Source: three-view drawing plus pictorial views. Frame: mm from the lowest corner of the part. Coordinates: 2 decimals unless noted, no trailing zeros. Loops run counter-clockwise (first coordinate to the right, second up) from the corner with the lowest first, then second, coordinate; pieces in that order, holes last.
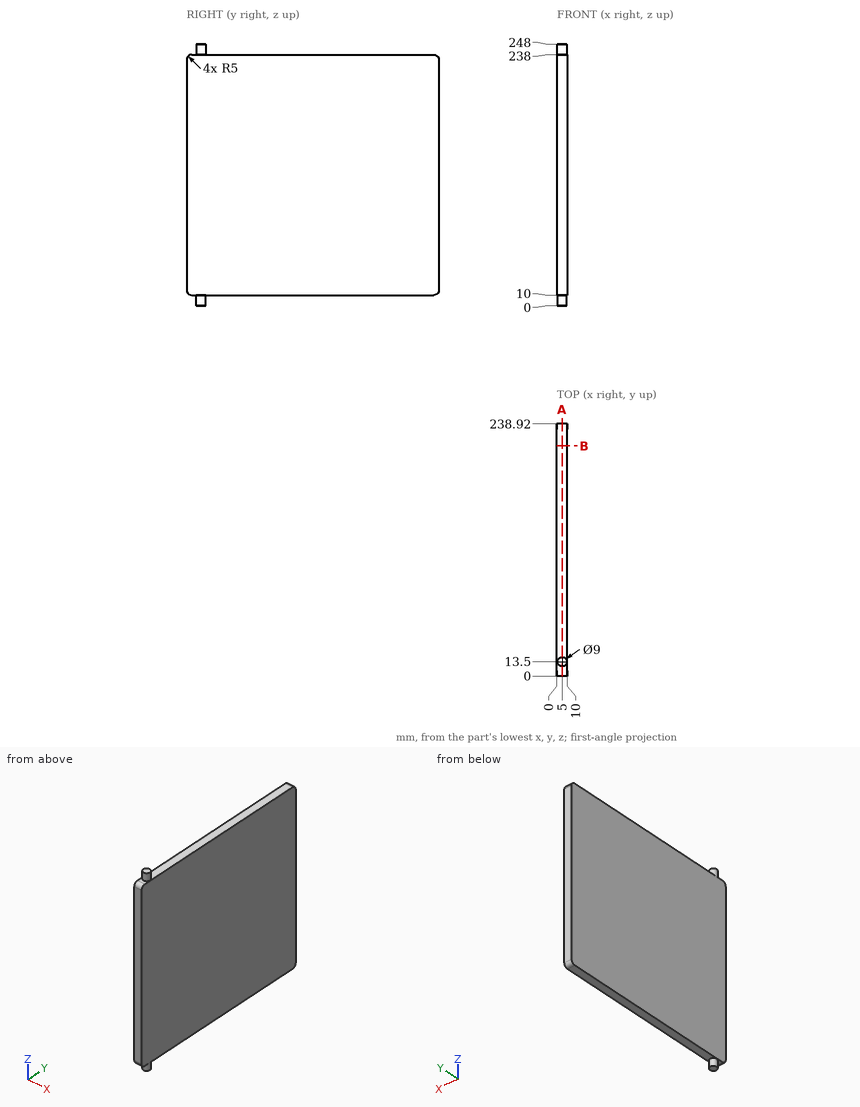
Q1. Section query A-A on x = 5. Return the cut outline in (y, z), then the cut area to 3 significant figures.
Q2. Material intervals for line 1 along Z through (x, y) = (7, 214), sorted ascending.
Q3. First-contact query: pin 1 Ø1 at (x, z) = (6.5, 139.5) entering from -Y; pin 2 Ø1 at (x, y) = (7, 87) entering from -Z; pin 3 Ø3 at (x, y) = (6.5, 103.5) entering from +Z. Flat tips, straight axial feed; report the tip coordinate or a pass-through.
Q4. Section query B-B on y = 218. Return the cut outline in (x, z), then the cut area to 3 significant figures.
Resolved:
1. outline: (0, 15) arc R5 ccw to (5, 10) - (9, 10) - (9, 0) - (18, 0) - (18, 10) - (233.92, 10) arc R5 ccw to (238.92, 15) - (238.92, 233) arc R5 ccw to (233.92, 238) - (18, 238) - (18, 248) - (9, 248) - (9, 238) - (5, 238) arc R5 ccw to (0, 233) - close
1. area: 54,600 mm2
2. line 1: z = 10 to 238
3. pin 1: stops at y = 0
3. pin 2: stops at z = 10
3. pin 3: stops at z = 238
4. outline: (0, 10) - (10, 10) - (10, 238) - (0, 238) - close
4. area: 2,280 mm2
